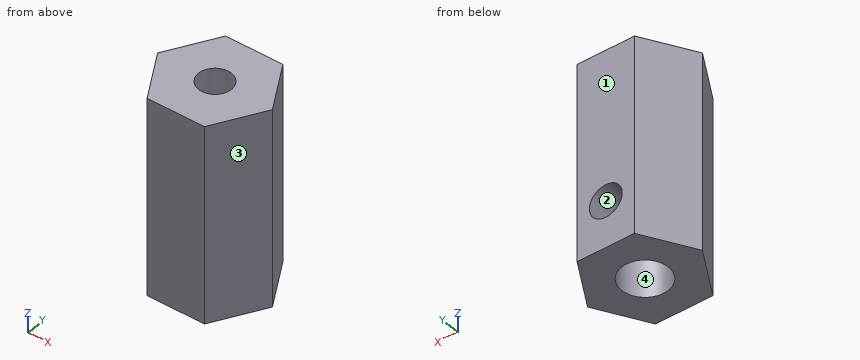
from build123d import *

# Parameters (mm, degrees)
BOSS_EXTRUDE1_DEPTH              = 25.4
SKETCH2_R                        = 3
CUT_EXTRUDE1_DEPTH               = 12.7
TAP_DRILL_FOR_M5X0_8_TAP1_D      = 4.2
TAP_DRILL_FOR_M5X0_8_TAP2_REACH  = 26.319
TAP_DRILL_FOR_M5X0_8_TAP2_BORE_R = 2.1


with BuildPart() as part:
    # Sketch1 → Boss-Extrude1 (new body)
    with BuildSketch(Plane.XY):
        Polygon((7.332348419, 0), (3.666174209, 6.35), (-3.666174209, 6.35), (-7.332348419, 0), (-3.666174209, -6.35), (3.666174209, -6.35), align=None)
    extrude(amount=BOSS_EXTRUDE1_DEPTH)

    # Sketch2 → Cut-Extrude1 (cut)
    with BuildSketch(Plane(origin=(0, 0, 0), x_dir=(-1, 0, 0), z_dir=(0, 0, -1))):
        Circle(SKETCH2_R)
    extrude(amount=-CUT_EXTRUDE1_DEPTH, mode=Mode.SUBTRACT)

    # Tap Drill for M5x0.8 Tap1 (through all)
    with Locations(Plane.XY.offset(25.4)):
        with Locations((0, 0)):
            Hole(TAP_DRILL_FOR_M5X0_8_TAP1_D / 2)

    # Tap Drill for M5x0.8 Tap2 bore (on position points) → Tap Drill for M5x0.8 Tap2 (cut, up to next)
    with BuildSketch(Plane(origin=(0, 6.35, 6), x_dir=(1, 0, 0), z_dir=(0, 1, 0)), mode=Mode.PRIVATE) as tap_drill_for_m5x0_8_tap2_sk1:
        Circle(TAP_DRILL_FOR_M5X0_8_TAP2_BORE_R)
    tap_drill_for_m5x0_8_tap2_tool1 = extrude(tap_drill_for_m5x0_8_tap2_sk1.sketch, amount=-TAP_DRILL_FOR_M5X0_8_TAP2_REACH, mode=Mode.PRIVATE) & part.part
    add(tap_drill_for_m5x0_8_tap2_tool1.solids().sort_by_distance((0, 6.35, 6))[0], mode=Mode.SUBTRACT)


solid = part.part
Work out the finished part from the listing and answer in its coordinate system (mm). Face numbers are marked on the shaded views. Give positions to 0.01 mm unless a question says otherwise; leave off trailing zeros. Loops run counter-clockwise (first coordinate to the right, second up) from the corner with the lowest first, then second, coordinate; pieces in that order, holes last. Notation, with made-up numbers: (14, 47.5) - (50, 47.5) arc R29 ccw to (50, 69.5) - close; hole circle Ø11 at (16, -0.75). An arc over 180 degrees is marked (long way). Answer in a Markdown table with one row per item. Add a question column.
Q1. The part is cut by section A-A (x = 0). Determine the outline of the cut face in (y, z).
Q2. The part is cut by section B-B (z = 2.75). Determine the outline of the cut face in (x, y).
Q3. The part is cut by section C-C (y = 1.75). Determine the outline of the cut face in (x, z), and give its area (3 significant figures).
Q4. Determine the mould class of the marked faces 1, 2, 3 and 4 for opening direction X: released by +X, released by -X, zero draft, split by the parting line, or undercut.
Q5. The part is cut by section D-D (z = 6). Determine the outline of the cut face in (x, y), and give its area (3 significant figures).
Q6. Each of these flat-tipped pins is pushed along its axis until it touches: P1, Ø1, axis at y = -3.5, z = 8.5, coming from the -X side; P2, Ø3, axis at x = -5, z = 3.5, coming from the +Y side; P3, Ø2.5, axis at x = 0, z = 6, coming from the +Y side; P4, Ø1.8, axis at x = 1, y = 0.5, coming from the -Z side. Where does it stop, or does it pass through?
Q7. Consider line 1 along Y through (x, z) = (0, 2.75); line 2 along Y through (x, z) = (0, 22.5); line 3 along Z through (x, y) = (1.5, 1.5). Determine where each line is inside the solid, lowest interval first.
Solution:
| question | item | result |
|---|---|---|
| 1 | outline | (-6.35, 0) - (-3, 0) - (-3, 12.7) - (-2.1, 12.7) - (-2.1, 25.4) - (-6.35, 25.4) - close; (2.1, 12.7) - (3, 12.7) - (3, 8.1) - (6.35, 8.1) - (6.35, 25.4) - (2.1, 25.4) - close; (3, 0) - (6.35, 0) - (6.35, 3.9) - (3, 3.9) - close |
| 2 | outline | (-7.33, 0) - (-3.67, -6.35) - (3.67, -6.35) - (7.33, 0) - (3.67, 6.35) - (-3.67, 6.35) - close; hole circle Ø6 at (0, 0) |
| 3 | outline | (-6.32, 0) - (-2.44, 0) - (-2.44, 12.7) - (-1.16, 12.7) - (-1.16, 25.4) - (-6.32, 25.4) - close; (1.16, 12.7) - (2.44, 12.7) - (2.44, 0) - (6.32, 0) - (6.32, 25.4) - (1.16, 25.4) - close |
| 3 | area | 230 mm² |
| 4 | face 1 | zero draft |
| 4 | face 2 | undercut |
| 4 | face 3 | released by +X |
| 4 | face 4 | undercut |
| 5 | outline | (-7.33, 0) - (-3.67, -6.35) - (3.67, -6.35) - (7.33, 0) - (3.67, 6.35) - (2.1, 6.35) - (2.1, 2.14) arc R3 cw (long way) to (-2.1, 2.14) - (-2.1, 6.35) - (-3.67, 6.35) - close |
| 5 | area | 96.2 mm² |
| 6 | P1 | stops at x = -5.6 |
| 6 | P2 | stops at y = 6.35 |
| 6 | P3 | stops at y = -2.73 |
| 6 | P4 | passes through |
| 7 | line 1 | y = -6.35 to -3, 3 to 6.35 |
| 7 | line 2 | y = -6.35 to -2.1, 2.1 to 6.35 |
| 7 | line 3 | z = 12.7 to 25.4 |
